Verification items for the finished model (mm, model axes). A direction names the side the tool comes from. Round coordinates to 2 decimals unless told otherwise and drop trailing zeros. Order: outer loops, then holes, each group sorted by start corner. A loop starts at its lowest first (then second) coordinate and runs counter-clockwise, first axis right, second up. Notation, with made-up numbers: M -9,64 L 1,64 A23 ccw 1,90 Z; hole C -39,32 d2. An arc over 180 degrees is marked long. One line per item, written item: value. Start each with the question number.
Solid Edge part; units mm, degrees
sketch "Sketch1" plane through (0, 0, 0) normal (0, 0, 1) x (1, 0, 0)
  line L0 (7.5, -60.5) -> (-7.5, -60.5)
  line L1 (-7.5, -60.5) -> (-7.5, -62.5)
  line L2 (-7.5, -62.5) -> (-17.5, -62.5)
  line L3 (-17.5, -62.5) -> (-17.5, -60.5)
  line L4 (-17.5, -60.5) -> (-39.5, -60.5)
  line L5 (-39.5, -60.5) -> (-39.5, 30.5)
  line L6 (-39.5, 30.5) -> (-17.5, 30.5)
  line L7 (-17.5, 30.5) -> (-17.5, 32.5)
  line L8 (-17.5, 32.5) -> (-7.5, 32.5)
  line L9 (-7.5, 32.5) -> (-7.5, 30.5)
  line L10 (-7.5, 30.5) -> (7.5, 30.5)
  line L11 (7.5, 30.5) -> (7.5, 32.5)
  line L12 (7.5, 32.5) -> (17.5, 32.5)
  line L13 (17.5, 32.5) -> (17.5, 30.5)
  line L14 (17.5, 30.5) -> (39.5, 30.5)
  line L15 (39.5, 30.5) -> (39.5, -60.5)
  line L16 (39.5, -60.5) -> (17.5, -60.5)
  line L17 (17.5, -60.5) -> (17.5, -62.5)
  line L18 (17.5, -62.5) -> (7.5, -62.5)
  line L19 (7.5, -62.5) -> (7.5, -60.5)
  line L20 (37.5, -45) -> (37.5, -35)
  line L21 (35.5, -45) -> (37.5, -45)
  line L22 (35.5, -35) -> (35.5, -45)
  line L23 (37.5, -35) -> (35.5, -35)
  line L24 (-35.5, -20) -> (-35.5, -10)
  line L25 (-37.5, -20) -> (-35.5, -20)
  line L26 (-37.5, -10) -> (-37.5, -20)
  line L27 (-35.5, -10) -> (-37.5, -10)
  line L28 (-37.5, -35) -> (-37.5, -45)
  line L29 (-35.5, -35) -> (-37.5, -35)
  line L30 (-35.5, -45) -> (-35.5, -35)
  line L31 (-37.5, -45) -> (-35.5, -45)
  line L32 (35.5, 5) -> (37.5, 5)
  line L33 (35.5, 15) -> (35.5, 5)
  line L34 (37.5, 15) -> (35.5, 15)
  line L35 (37.5, 5) -> (37.5, 15)
  circle A0 centre (32.96, -12.96) radius 1.3
  circle A1 centre (32.96, -57.96) radius 1.3
  line L36 (-37.5, 5) -> (-35.5, 5)
  line L37 (-37.5, 15) -> (-37.5, 5)
  line L38 (-35.5, 15) -> (-37.5, 15)
  line L39 (-35.5, 5) -> (-35.5, 15)
  line L40 (35.5, -10) -> (35.5, -20)
  line L41 (37.5, -10) -> (35.5, -10)
  line L42 (37.5, -20) -> (37.5, -10)
  line L43 (35.5, -20) -> (37.5, -20)
extrude "ExtrudedProtrusion_1" add sketch "Sketch1" along normal blind 2
properties material "Acrylic, high impact grade"
1. Draft check along X on faces 1 (the face through (-29, 30.5, 1)), 2 (the face through (7.5, -62, 1)), 3 (the face through (32.002, -58.839, 0.986)), 4 (the face through (17.5, 32, 1)). Enter one of: released by +X, released by -X, zero draft, split by the parting line, or undercut.
2. Section check A-A (y = -12.96). Record the cut outline in (x, z), and give its area (3 significant figures).
3. Scan lines: line 1 along Y through (x, z) = (32.96, 0.45); line 2 along X through (y, z) = (-16, 0.4); line 3 along Y through (x, z) = (-2, 0.8). Record each from-to range of solid material in increasing order.
4. Section check C-C (y = -57.96). Record the cut outline in (x, z), and give its area (3 significant figures).
5. Tool access check on faces 5 (the face through (-35.5, -15, 1)), 6 (the face through (-28, -60.5, 1)), 7 (the face through (-17.5, 31, 1)), 8 (the face through (29, -60.5, 1)). Record the directions out of +Z, -Z, +X, -X, +Y, -Y that give a thin tool (end or side, any length) a straight path to the whole face; none if there is none.
6. Depth check by flat-ended pin: pin 1 (1 mm diameter, centred on y = -61.5, z = 0.5, fed in from -X); pin 2 (0.6 mm diameter, centred on y = -61.5, z = 1.5, fed in from +X); pin 3 (1 mm diameter, centred on x = -37, z = 1, fed in from +Y). Enter the tip coordinate at first touch or a pass-through.
7. Section check D-D (y = 10.5). Record the cut outline in (x, z), and give its area (3 significant figures).
8. Section check B-B (x = 32.96). Record the cut outline in (y, z), and give its area (3 significant figures).
Geometry check:
1. face 1: zero draft
1. face 2: undercut
1. face 3: undercut
1. face 4: released by +X
2. outline: M -39.5,0 L -37.5,0 L -37.5,2 L -39.5,2 Z; M -35.5,0 L 31.66,0 L 31.66,2 L -35.5,2 Z; M 34.26,0 L 35.5,0 L 35.5,2 L 34.26,2 Z; M 37.5,0 L 39.5,0 L 39.5,2 L 37.5,2 Z
2. area: 145 mm²
3. line 1: y = -60.5 to -59.26, -56.66 to -14.26, -11.66 to 30.5
3. line 2: x = -39.5 to -37.5, -35.5 to 35.5, 37.5 to 39.5
3. line 3: y = -60.5 to 30.5
4. outline: M -39.5,0 L 31.66,0 L 31.66,2 L -39.5,2 Z; M 34.26,0 L 39.5,0 L 39.5,2 L 34.26,2 Z
4. area: 153 mm²
5. face 5: +Z, -Z
5. face 6: +Z, -Z, -X, -Y
5. face 7: +Z, -Z, -X, +Y
5. face 8: +Z, -Z, +X, -Y
6. pin 1: stops at x = -17.5
6. pin 2: stops at x = 17.5
6. pin 3: stops at y = 30.5
7. outline: M -39.5,0 L -37.5,0 L -37.5,2 L -39.5,2 Z; M -35.5,0 L 35.5,0 L 35.5,2 L -35.5,2 Z; M 37.5,0 L 39.5,0 L 39.5,2 L 37.5,2 Z
7. area: 150 mm²
8. outline: M -60.5,0 L -59.26,0 L -59.26,2 L -60.5,2 Z; M -56.66,0 L -14.26,0 L -14.26,2 L -56.66,2 Z; M -11.66,0 L 30.5,0 L 30.5,2 L -11.66,2 Z
8. area: 172 mm²
